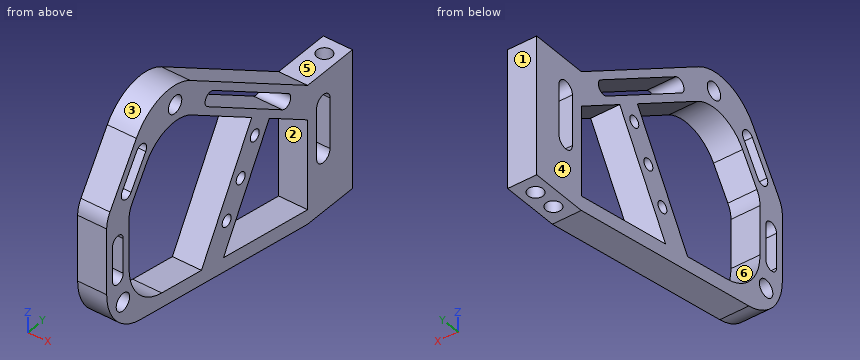
from build123d import *

# Parameters (mm, degrees)
SKETCH_R        = 1.5
SKETCH_R_2      = 1
PAD_DEPTH       = 2.5
SKETCH002_R     = 1.3
POCKET001_DEPTH = 5
SKETCH003_R     = 1.3
POCKET002_DEPTH = 5


with BuildPart() as part:
    # Sketch → Pad (new body, symmetric)
    with BuildSketch(Plane.YZ):
        with BuildLine():
            Line((5, -12), (-5, -12))
            Line((-5, -12), (-42.491034, -5.389319))
            ThreePointArc((-50, 3.559518), (-47.874072, -2.281421), (-42.491034, -5.389319))
            Line((-50, 3.559518), (-50, 14.930703))
            ThreePointArc((-49.265951, 17.408811), (-49.81263, 16.222973), (-50, 14.930703))
            Line((-49.265951, 17.408811), (-43.362064, 26.5))
            ThreePointArc((-31.281961, 29.067705), (-37.853802, 30.285724), (-43.362064, 26.5))
            Line((-5, 12), (-31.281961, 29.067705))
            Line((5, 12), (-5, 12))
            Line((5, 12), (5, -9.5))
            Line((5, -12), (5, -9.5))
        make_face()
        with Locations((-34.683969, 26.982892)):
            Circle(SKETCH_R, mode=Mode.SUBTRACT)
        with Locations((-46.364789, 0.041977)):
            Circle(SKETCH_R, mode=Mode.SUBTRACT)
        with Locations((-20, 5.209335)):
            Circle(SKETCH_R_2, mode=Mode.SUBTRACT)
        with Locations((-16.855, 10.656635)):
            Circle(SKETCH_R_2, mode=Mode.SUBTRACT)
        with Locations((-23.145, -0.237965)):
            Circle(SKETCH_R_2, mode=Mode.SUBTRACT)
        Polygon((-5, 6.038184), (-5, -9.5), (-23.859805, -6.174507), (-13.588624, 11.615701), align=None, mode=Mode.SUBTRACT)
        with BuildLine():
            Line((-41.094301, 20.811657), (-44.299169, 15.876592))
            ThreePointArc((-44.299169, 15.876592), (-44.821109, 14.744417), (-45, 13.510627))
            Line((-45, 13.510627), (-45, 5))
            ThreePointArc((-45, 5), (-42.923669, -0.704672), (-37.666214, -3.740065))
            Line((-37.666214, -3.740065), (-28.783844, -5.306267))
            Line((-17.534494, 14.178179), (-28.783844, -5.306267))
            Line((-31.040008, 22.948763), (-17.534494, 14.178179))
            ThreePointArc((-31.040008, 22.948763), (-36.509764, 23.962522), (-41.094301, 20.811657))
        make_face(mode=Mode.SUBTRACT)
        with BuildLine():
            ThreePointArc((-26.119845, 24.165315), (-27.779816, 23.812477), (-27.426978, 22.152506))
            Line((-27.426978, 22.152506), (-10.653567, 11.259725))
            ThreePointArc((-10.653567, 11.259725), (-8.993595, 11.612563), (-9.346433, 13.272534))
            Line((-26.119845, 24.165315), (-9.346433, 13.272534))
        make_face(mode=Mode.SUBTRACT)
        with BuildLine():
            ThreePointArc((-46.541762, 19.216792), (-46.188924, 17.55682), (-44.528953, 17.909658))
            Line((-44.528953, 17.909658), (-41.261119, 22.941682))
            ThreePointArc((-41.261119, 22.941682), (-41.613957, 24.601653), (-43.273928, 24.248815))
            Line((-46.541762, 19.216792), (-43.273928, 24.248815))
        make_face(mode=Mode.SUBTRACT)
        with BuildLine():
            ThreePointArc((-46.3, 11), (-47.5, 12.2), (-48.7, 11))
            Line((-48.7, 11), (-48.7, 5))
            ThreePointArc((-48.7, 5), (-47.5, 3.8), (-46.3, 5))
            Line((-46.3, 11), (-46.3, 5))
        make_face(mode=Mode.SUBTRACT)
        with BuildLine():
            ThreePointArc((0, 6.746165), (-1.5, 8.246165), (-3, 6.746165))
            Line((-3, 6.746165), (-3, -2))
            ThreePointArc((-3, -2), (-1.5, -3.5), (0, -2))
            Line((0, 6.746165), (0, -2))
        make_face(mode=Mode.SUBTRACT)
    extrude(amount=PAD_DEPTH, both=True)

    # Sketch002 (on Face9 of Pad) → Pocket001 (cut)
    with BuildSketch(Plane(origin=(0, 0, 12), x_dir=(0, -1, 0), z_dir=(0, 0, 1))):
        with Locations((-2, 0)):
            Circle(SKETCH002_R)
    extrude(amount=-POCKET001_DEPTH, mode=Mode.SUBTRACT)

    # Sketch003 (on Face1 of Pocket001) → Pocket002 (cut)
    with BuildSketch(Plane.YX.offset(12)):
        with Locations((-2, 0)):
            Circle(SKETCH003_R)
        with Locations((2, 0)):
            Circle(SKETCH003_R)
    extrude(amount=-POCKET002_DEPTH, mode=Mode.SUBTRACT)


solid = part.part
CAD build for the part. Positions are in the model's coordinates, mm. Face numbers are marked on the shaded views. A direction names the side the tool comes from. Give positions to 0.01 mm unless a question says otherwise; leave off trailing zeros. Loops run counter-clockwise (first coordinate to the right, second up) from the corner with the lowest first, then second, coordinate; pieces in that order, holes last. Notation, with made-up numbers: M -27.75,-22 L 11.25,-22 A11 ccw 11.25,-7 Z; hole C 23.25,-25.75 d6. An arc over 180 degrees is marked long. One line per question, with ' | ' between items. Start each with the question number.
1. Saw through at B-B on y = -16.5. Give the cut face in (x, z), plus the area to 3 significant figures.
2. 3-axis set-ups, long thin cutter, end or side, ignore diameter. For the marked faces 4, 5 and 6: which of +Z, -Z, +X, -X, +Y, -Y reach the whole face in a straight line?
3. Two-plate mould, pull along Z, no slides. Class the marked faces 1, 2 and 3: pulls with the +Z half, pulls with the -Z half, needs draft (parallel to the pull), parting line crosses it, or undercut.
4. Saw through at C-C on x = 1.9. State how many separate pieces and enclosed holes the cut face has, plus the area to 3 significant figures.
5. Probe L1, parallel to Z at x = -1.3, y = -17; L2, parallel to Y at x = -0.55, z = 18; L3, parallel to Z at x = -0.05, y = -23. List the from-to ranges inside material, lowest first. Write a range as from..to.
6. Saw through at A-A on y = -1.5. Give the cut face in (x, z).
7. Flat gauge pins, fed straight in: pin 1 (3 mm diameter, centred on x = -0.5, y = 2, fed in from +Z); pin 2 (2 mm diameter, centred on x = 0, y = -2, fed in from -Z); pin 3 (2 mm diameter, centred on x = 0, y = 2, fed in from +Z). Where does each tip first touch, or does it go through?
Result sheet:
1) outline: M -2.5,-9.97 L 2.5,-9.97 L 2.5,-7.47 L -2.5,-7.47 Z; M -2.5,6.57 L 2.5,6.57 L 2.5,9.72 L -2.5,9.72 Z; M -2.5,11.59 L 2.5,11.59 L 2.5,15.06 L -2.5,15.06 Z; M -2.5,17.92 L 2.5,17.92 L 2.5,19.47 L -2.5,19.47 Z | area: 53.3 mm^2
2) face 4: +Z, -Z, -X, +Y, -Y | face 5: +Z, +X, -X, +Y | face 6: +X, -X
3) face 1: needs draft | face 2: undercut | face 3: pulls with the +Z half
4) separate pieces: 1 | enclosed holes: 11 | area: 673 mm^2
5) L1: z = -9.88..-7.38, 5.71..9.67, 11.65..15.38, 18.24..19.79 | L2: y = -48.88..-46.59, -44.47..-42.92, -23.42..-21.03, -16.63..-14.24 | L3: z = -8.83..-6.33, -4.69..-1.23, 0.75..4.71, 17.73..19.28, 22.14..23.69
6) outline: M -2.5,-12 L -1.2,-12 L -1.2,-7 L 1.2,-7 L 1.2,-12 L 2.5,-12 L 2.5,-3.5 L -2.5,-3.5 Z; M -2.5,8.25 L 2.5,8.25 L 2.5,12 L -2.5,12 Z
7) pin 1: stops at z = 12 | pin 2: stops at z = -7 | pin 3: stops at z = 7
